from build123d import *

# Parameters (mm, degrees)
F0_R     = 8.4375
F1_DEPTH = 12.7
F2_R     = 6.34999
F3_R     = 2.88125
F4_DEPTH = 25.401


# Not quite as in the source:
# - a fillet or chamfer is up to 0.001 mm smaller than in the source, because OpenCascade refuses the exact size


with BuildPart() as f1:
    # F0 (on Front) → F1 (new body)
    with BuildSketch(Plane.XZ):
        with BuildLine():
            ThreePointArc((0, -12.7), (-8.9802561211, -8.9802561211), (-12.7, 0))
            Line((-12.7, 0), (-12.7, -25.4))
            Line((-12.7, -25.4), (-6.35, -25.4))
            Line((-6.35, -25.4), (-6.35, -12.7))
            Line((-6.35, -12.7), (0, -12.7))
        make_face()
        with BuildLine():
            Line((12.7, -25.4), (12.7, 0))
            ThreePointArc((12.7, 0), (8.9802561211, -8.9802561211), (0, -12.7))
            Line((0, -12.7), (6.35, -12.7))
            Line((6.35, -12.7), (6.35, -25.4))
            Line((6.35, -25.4), (12.7, -25.4))
        make_face()
        with BuildLine():
            ThreePointArc((0, -12.7), (8.9802561211, -8.9802561211), (12.7, 0))
            ThreePointArc((12.7, 0), (0, 12.7), (-12.7, 0))
            ThreePointArc((-12.7, 0), (-8.9802561211, -8.9802561211), (0, -12.7))
        make_face()
        Circle(F0_R, mode=Mode.SUBTRACT)
    extrude(amount=F1_DEPTH)

    # F2 (radius 6.35 in the source; OpenCascade refuses exactly that, so slightly less here)
    f2_edges = [f1.edges().sort_by_distance(p)[0] for p in [
        (-9.525, -12.7, -25.4),
        (-9.525, 0, -25.4),
        (9.525, -12.7, -25.4),
        (9.525, 0, -25.4),
    ]]
    fillet(f2_edges, radius=F2_R)

    # F3 (on face) → F4 (cut, through all)
    with BuildSketch(Plane.YZ.offset(12.7)):
        with Locations((-6.35, -19.05)):
            Circle(F3_R)
    extrude(amount=-F4_DEPTH, mode=Mode.SUBTRACT)


solid = f1.part
The listing builds one solid part. Answer for the finished solid, in the listing's coordinates (mm). A direction names the side the tool comes from. Coordinates: 2 decimals unless noted, no trailing zeros. Write each loop counter-clockwise with the first axis right and the second up, starting at its lowest first coordinate (ties: lowest second). Pieces come first, ordered by that corner, then holes. Notation, with made-up numbers: (36.25, -33.5) - (56.25, -33.5) arc R23 cw to (56.25, 3.5) - close; hole circle Ø11 at (43, 41). An arc over 180 degrees is marked (long way). Return JSON: item names as keys, results as strings.
1. Which of the six approach directions +Z, -Z, +X, -X, +Y, -Y give full straight-line access (tool end or side, diameter ignored) to faces 4 (the face through (-9.48, -10.79, -23.59)), 5 (the face through (-6.35, -8, -16))?
Final values:
{"face 4": "-Z, +X, -X, -Y", "face 5": "-Z, +Y, -Y"}
2. The part is cut by section C-C on x = 0. Determine the outline of the cut face in (y, z), then the cut area to 3 significant figures.
Final values:
{"outline": "(-12.7, -12.7) - (0, -12.7) - (0, -8.44) - (-12.7, -8.44) - close; (-12.7, 8.44) - (0, 8.44) - (0, 12.7) - (-12.7, 12.7) - close", "area": "108 mm^2"}
3. The part is cut by section B-B on y = -8.5. Count the separate pieces of the cut face and the enclosed holes in it, then the cut area to 3 significant figures.
Final values:
{"separate pieces": "3", "enclosed holes": "1", "area": "460 mm^2"}
4. The part is cut by section A-A on z = -14.5. Determine the outline of the cut face in (x, y).
Final values:
{"outline": "(-12.7, -12.7) - (-6.35, -12.7) - (-6.35, 0) - (-12.7, 0) - close; (6.35, -12.7) - (12.7, -12.7) - (12.7, 0) - (6.35, 0) - close"}
5. For a pull along Z with two mould halves and no side action, classify faces 1 (the face through (0.279, -6.261, 12.697)), 2 (the face through (-5.8, -12.7, -6.5)), 3 (the face through (-9.48, -9.23, -18.92)) as +Z half, -Z half, draft (parallel to the pull), parting line (faces both ways), or undercut.
Final values:
{"face 1": "+Z half", "face 2": "draft", "face 3": "undercut"}
6. Each of these flat-tipped pins is pushed along its axis until it touches: pin 1 Ø1 at (x, z) = (-8.5, 6.5) entering from +Y; pin 2 Ø4 at (x, y) = (-2, -5) entering from -Z; pin 3 Ø3.5 at (y, z) = (-6.35, -19.05) entering from +X; pin 4 Ø2 at (x, y) = (1.5, -5) entering from +Z. Where does it stop, or does it pass through?
Final values:
{"pin 1": "y = 0", "pin 2": "z = -12.7", "pin 3": "through", "pin 4": "z = 12.69"}
7. Consider line 1 along X through (y, z) = (-9.75, -13); line 2 along Z through (x, y) = (11, -6.35); line 3 along Z through (x, y) = (0, -2.5). Determine where each line is inside the solid, lowest interval first.
Final values:
{"line 1": "-12.7 to -6.35, 6.35 to 12.7", "line 2": "-25.4 to -21.93, -16.17 to 6.35", "line 3": "-12.7 to -8.44, 8.44 to 12.7"}
